Source: three-view drawing plus pictorial views. Frame: mm from the lowest corner of the part. Give positions to 0.01 mm unless a question says otherwise; leave off trailing zeros. Loops run counter-clockwise (first coordinate to the right, second up) from the corner with the lowest first, then second, coordinate; pieces in that order, holes last. Notation, with made-up numbers: (78, 72) - (95, 72) arc R28 ccw to (95, 104) - close; hole circle Ø9 at (44, 77.25). An arc over 180 degrees is marked (long way). Answer in a Markdown table with one row per item.
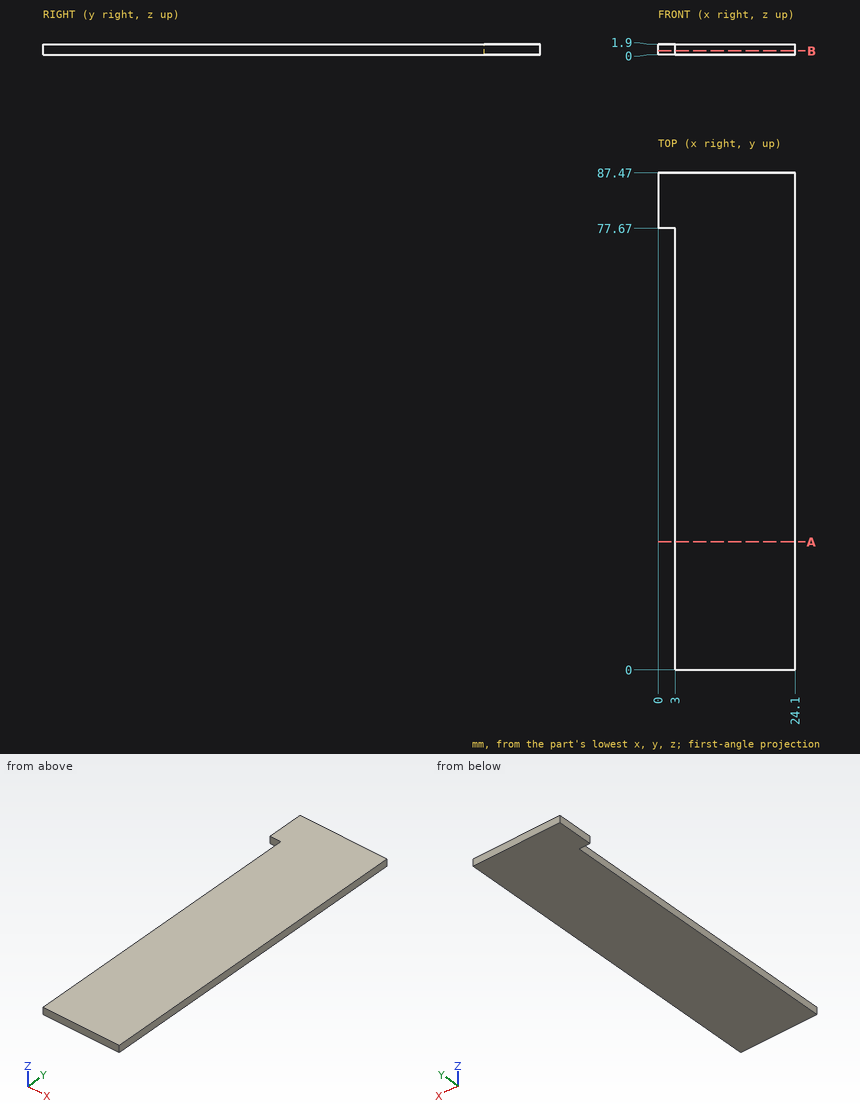
Q1. Material intervals for line 1 along X through (y, z) = (68, 0.7); line 2 along Y through (x, z) = (2.75, 0.5), sorted ascending.
Check values:
| item | result |
|---|---|
| line 1 | 3 to 24.1 |
| line 2 | 77.67 to 87.47 |
Q2. Cut plane A-A (y = 22.5). Output: boundary loops of the cut face in (x, z), and give its area (3 significant figures).
Check values:
| item | result |
|---|---|
| outline | (3, 0) - (24.1, 0) - (24.1, 1.9) - (3, 1.9) - close |
| area | 40.1 mm² |
Q3. Cut plane B-B (z = 0.7). Output: boundary loops of the cut face in (x, y), and give its area (3 significant figures).
Check values:
| item | result |
|---|---|
| outline | (0, 77.67) - (3, 77.67) - (3, 0) - (24.1, 0) - (24.1, 87.47) - (0, 87.47) - close |
| area | 1,880 mm² |
